Geometry: final body of the model. Coordinates: model frame, mm. Face numbers are marked on the shaded views. Give positions to 0.01 mm unless a question says otherwise; leave off trailing zeros. Loops run counter-clockwise (first coordinate to the right, second up) from the corner with the lowest first, then second, coordinate; pieces in that order, holes last.
```python
from build123d import *

# Parameters (mm, degrees)
SKETCH1_W                       = 40
SKETCH1_H                       = 52
SKETCH1_R                       = 14
BOSS_EXTRUDE1_DEPTH             = 20
M5X0_8_TAPPED_HOLE1_D           = 4.2
M5X0_8_TAPPED_HOLE1_DEPTH       = 10
M5X0_8_TAPPED_HOLE1_CSINK_D     = 5.05
M5X0_8_TAPPED_HOLE1_CSINK_ANGLE = 90
M5X0_8_TAPPED_HOLE1_TIP         = 1.2618073
CHAMFER1_SIZE                   = 12
M5X0_8_TAPPED_HOLE2_D           = 4.2
M5X0_8_TAPPED_HOLE2_DEPTH       = 12.4
M5X0_8_TAPPED_HOLE2_CSINK_D     = 5.05
M5X0_8_TAPPED_HOLE2_CSINK_ANGLE = 90
M5X0_8_TAPPED_HOLE2_TIP         = 1.2618073


with BuildPart() as part:
    # Sketch1 → Boss-Extrude1 (new, symmetric)
    with BuildSketch(Plane.XY):
        Rectangle(SKETCH1_W, SKETCH1_H)
        Circle(SKETCH1_R, mode=Mode.SUBTRACT)
    extrude(amount=BOSS_EXTRUDE1_DEPTH, both=True)

    # M5x0.8 Tapped Hole1
    with Locations(Plane.XY.offset(20)):
        with Locations((-13.435028843, 13.435028843), (0, 19), (13.435028843, 13.435028843), (13.435028843, -13.435028843), (0, -19), (-13.435028843, -13.435028843)):
            CounterSinkHole(M5X0_8_TAPPED_HOLE1_D / 2, M5X0_8_TAPPED_HOLE1_CSINK_D / 2, depth=M5X0_8_TAPPED_HOLE1_DEPTH, counter_sink_angle=M5X0_8_TAPPED_HOLE1_CSINK_ANGLE)
            with Locations((0, 0, -(M5X0_8_TAPPED_HOLE1_DEPTH + M5X0_8_TAPPED_HOLE1_TIP / 2))):  # 118° drill point
                Cone(0, M5X0_8_TAPPED_HOLE1_D / 2, M5X0_8_TAPPED_HOLE1_TIP, mode=Mode.SUBTRACT)

    # Chamfer1
    chamfer1_edges = [part.edges().sort_by_distance(p)[0] for p in [
        (-20, -26, 0),
        (-20, 26, 0),
    ]]
    chamfer(chamfer1_edges, length=CHAMFER1_SIZE)

    # M5x0.8 Tapped Hole2
    with Locations(Plane(origin=(20, 0, 0), x_dir=(0, 0, -1), z_dir=(1, 0, 0))):
        with Locations((-12, 20), (12, 20), (12, -20), (-12, -20)):
            CounterSinkHole(M5X0_8_TAPPED_HOLE2_D / 2, M5X0_8_TAPPED_HOLE2_CSINK_D / 2, depth=M5X0_8_TAPPED_HOLE2_DEPTH, counter_sink_angle=M5X0_8_TAPPED_HOLE2_CSINK_ANGLE)
            with Locations((0, 0, -(M5X0_8_TAPPED_HOLE2_DEPTH + M5X0_8_TAPPED_HOLE2_TIP / 2))):  # 118° drill point
                Cone(0, M5X0_8_TAPPED_HOLE2_D / 2, M5X0_8_TAPPED_HOLE2_TIP, mode=Mode.SUBTRACT)


solid = part.part
```
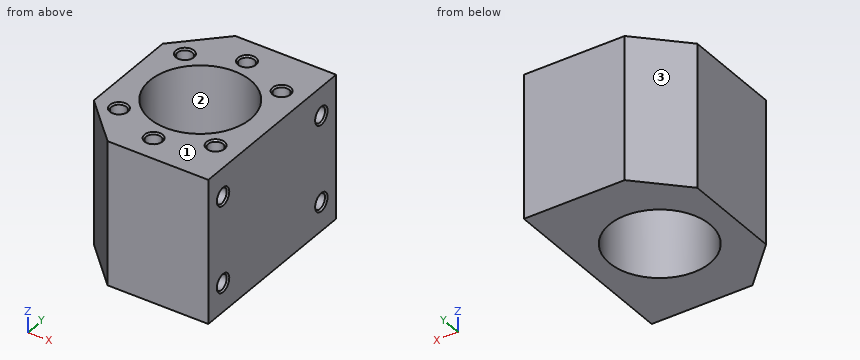
Q1. Pin query (flat end, axial travel): pin 1 Ø22.5 at (x, y) = (0, 0) entering from -Z; pin 2 Ø2.5 at (x, y) = (-13.44, -13.44) entering from +Z; pin 3 Ø5 at (y, z) = (20, -12) entering from +X (3 decimals); pin 4 Ø2.5 at (y, z) = (20, 12) entering from +X. Return the tip coordinate at first contact, or that it passes through.
Q2. Section query A-A, the plane y = 0. Return loops of the section in (x, z), and give its area (3 significant figures).
Q3. Section query C-C, the plane x = 4. Return loops of the section in (y, z), and give its area (3 significant figures).
Q4. Section query D-D, the plane z = 16. Return loops of the section in (x, y).
Q5. Section query B-B, the plane z = 4.5. Return loops of the section in (x, y), and give its area (3 significant figures).
Q6. Material intervals for probe 1 along Z at (x, y) = (16, -20); probe 2 along Y at (x, z) = (0, 13); probe 3 along Y at (x, z) = (0.5, 9), sorted ascending.
Q7. Mould query, pull axis Y, two halves, no side actions, for the marked faces 1, 2 and 3. Classes: +Y half, -Y half, draft (parallel to the pull), parting line (faces both ways), or undercut.
Resolved:
1. pin 1: passes through
1. pin 2: stops at z = 9.49
1. pin 3: stops at x = 19.975
1. pin 4: stops at x = 7.09
2. outline: (-20, -20) - (-14, -20) - (-14, 20) - (-20, 20) - close; (14, -20) - (20, -20) - (20, 20) - (14, 20) - close
2. area: 480 mm2
3. outline: (-26, -20) - (-13.42, -20) - (-13.42, 20) - (-26, 20) - close; (13.42, -20) - (26, -20) - (26, 20) - (13.42, 20) - close
3. area: 1,010 mm2
4. outline: (-20, -14) - (-8, -26) - (20, -26) - (20, 26) - (-8, 26) - (-20, 14) - close; hole circle Ø4.2 at (-13.44, -13.44); hole circle Ø4.2 at (-13.44, 13.44); hole circle Ø28 at (0, 0); hole circle Ø4.2 at (0, -19); hole circle Ø4.2 at (0, 19); hole circle Ø4.2 at (13.44, -13.44); hole circle Ø4.2 at (13.44, 13.44)
5. outline: (-20, -14) - (-8, -26) - (20, -26) - (20, 26) - (-8, 26) - (-20, 14) - close; hole circle Ø28 at (0, 0)
5. area: 1,320 mm2
6. probe 1: z = -20 to -14.1, -9.9 to 9.9, 14.1 to 20
6. probe 2: y = -26 to -21.1, -16.9 to -14, 14 to 16.9, 21.1 to 26
6. probe 3: y = -26 to -13.99, 13.99 to 26
7. face 1: draft
7. face 2: undercut
7. face 3: +Y half
